from build123d import *

# Parameters (mm, degrees)
BOSS_EXTRUDE1_DEPTH = 10
SKETCH3_R           = 2
BOSS_EXTRUDE2_DEPTH = 10
BOSS_EXTRUDE3_DEPTH = 20
SKETCH6_R           = 2
CUT_EXTRUDE2_DEPTH  = 20
SKETCH4_W           = 40
SKETCH4_H           = 10
CUT_EXTRUDE1_DEPTH  = 31.090136351
FILLET1_R           = 2


with BuildPart() as part:
    # Sketch1 → Boss-Extrude1 (new, symmetric)
    with BuildSketch(Plane(origin=(0, 0, 0), x_dir=(1, 0, 0), z_dir=(0, 1, 0))):
        Polygon((0, -4), (0, 18), (-17.5, 18), (-17.5, 22), (6, 22), (6, -4), align=None)
    extrude(amount=BOSS_EXTRUDE1_DEPTH, both=True)

    # Sketch3 → Boss-Extrude2 (add, symmetric)
    with BuildSketch(Plane(origin=(0, 0, 0), x_dir=(1, 0, 0), z_dir=(0, 1, 0))):
        with BuildLine():
            Line((-3, 4), (0, 4))
            Line((0, 4), (0, -4))
            Line((0, -4), (-3, -4))
            ThreePointArc((-3, -4), (-7, 0), (-3, 4))
        make_face()
        with Locations(Location((-3, 0, 0), (0, 0, 270))):
            Circle(SKETCH3_R, mode=Mode.SUBTRACT)
    extrude(amount=BOSS_EXTRUDE2_DEPTH, both=True)

    # Sketch5 → Boss-Extrude3 (add)
    with BuildSketch(Plane(origin=(0, 10, 0), x_dir=(1, 0, 0), z_dir=(0, 1, 0))):
        with BuildLine():
            Line((0, -4), (10.949747468, -14.949747468))
            ThreePointArc((10.949747468, -14.949747468), (16.606601718, -14.949747468), (16.606601718, -9.292893219))
            Line((16.606601718, -9.292893219), (6, 1.313708499))
            Line((6, 1.313708499), (0, -4))
        make_face()
    extrude(amount=-BOSS_EXTRUDE3_DEPTH)

    # Sketch6 → Cut-Extrude2 (cut)
    with BuildSketch(Plane(origin=(0, 10, 0), x_dir=(1, 0, 0), z_dir=(0, 1, 0))):
        with Locations(Location((13.778174593, -12.121320344, 0), (0, 0, 270))):
            Circle(SKETCH6_R)
    extrude(amount=-CUT_EXTRUDE2_DEPTH, mode=Mode.SUBTRACT)

    # Sketch4 → Cut-Extrude1 (cut, through all)
    with BuildSketch(Plane.XY.offset(-6)):
        with Locations((2.5, 0)):
            Rectangle(SKETCH4_W, SKETCH4_H)
    extrude(amount=CUT_EXTRUDE1_DEPTH, mode=Mode.SUBTRACT)

    # Fillet1
    fillet1_edges = [part.edges().sort_by_distance(p)[0] for p in [
        (6, 7.5, -1.313708499),
        (6, -7.5, -1.313708499),
        (0, -7.5, 4),
        (0, 7.5, 4),
        (0, 0, -18),
        (0, -7.5, -4),
        (0, 7.5, -4),
    ]]
    fillet(fillet1_edges, radius=FILLET1_R)


solid = part.part
Source: CAD feature listing. Evaluate the final solid. Frame: model axes, mm. A direction names the side the tool comes from. Coordinates: 2 decimals unless noted, no trailing zeros. Order: outer loops, then holes, each group sorted by start corner. A loop starts at its lowest first (then second) coordinate and runs counter-clockwise, first axis right, second up. Notation, with made-up numbers: M 63.5,9 L 87.5,9 A21 ccw 87.5,30 Z; hole C 4.5,3 d8. An arc over 180 degrees is marked long. Write each question's results on one line, items separated by ' | '. Start each with the question number.
Item 1: Cut plane A-A (y = -2.5). Return loops of the section in (x, z).
Item 2: Cut plane B-B (z = 0). Return loops of the section in (x, y), and give its area (3 significant figures).
Item 3: Set-up query: faces 5 (the face through (14.38, -7.46, 14.03)), 6 (the face through (-2, 8, 4)), 7 (the face through (11.666, 7.535, 4.353)), 8 (the face through (5, 5, 5)), 9 (the face through (-0.6, 7.46, -4.57)). Return all of +Z, -Z, +X, -X, +Y, -Y with unobstructed straight access to the full face (end or side cutting, diameter ignored); none if empty.
Item 4: Draft query along Z for faces 1 (the face through (0, 0, -11)), 2 (the face through (14.38, 7.54, 14.03)), 3 (the face through (1, -10, -6)), 4 (the face through (3, 0, -6)). Return one class per face: pulls with the +Z half, pulls with the -Z half, needs draft (parallel to the pull), parting line crosses it, or undercut.
Item 5: Line query: probe 1 along Z at (x, y) = (-3, -8.1); probe 2 along Y at (x, z) = (0, 1); probe 3 along Z at (x, y) = (-4.5, -1.5). Output: solid intervals per line, ascending.
Item 6: First-contact query: pin 1 Ø8 at (x, y) = (-12.5, -3.5) entering from +Z; pin 2 Ø1.8 at (x, y) = (1.5, -2.5) entering from +Z; pin 3 Ø10 at (y, z) = (-2.5, 6.5) entering from +X. Flat tips, straight axial feed; report the tip coordinate or a pass-through.
Item 7: Cut plane D-D (y = -8.25). Return loops of the section in (x, z).
Item 8: Cut plane C-C (x = 5.5). Return loops of the section in (y, z), and give its area (3 significant figures).
Checked values:
1) outline: M -17.5,-22 L 6,-22 L 6,-6 L 0,-6 L 0,-16 A2 cw -2,-18 L -17.5,-18 Z
2) outline: M -7,-10 L -5,-10 L -5,-5 L -7,-5 Z; M -7,5 L -5,5 L -5,10 L -7,10 Z; M -1,-10 L 7.31,-10 L 7.31,-5 L -1,-5 Z; M -1,5 L 7.31,5 L 7.31,10 L -1,10 Z | area: 103 mm2
3) face 5: +Y, -Y | face 6: +Z, -X, +Y, -Y | face 7: -Z, +X, +Y, -Y | face 8: +Z, +X, -X | face 9: -X, +Y, -Y
4) face 1: undercut | face 2: undercut | face 3: needs draft | face 4: pulls with the +Z half
5) probe 1: z = -22 to -18, -4 to -2, 2 to 4 | probe 2: y = -10 to -5, 5 to 10 | probe 3: z = -22 to -18
6) pin 1: stops at z = -18 | pin 2: stops at z = -6 | pin 3: stops at x = 17.56
7) outline: M -17.5,-22 L 6,-22 L 6,-2.14 A2 cw 6.59,-0.73 L 16.61,9.29 A4 ccw 10.95,14.95 L 0.59,4.59 A2 cw -0.83,4 L -3,4 A4 ccw -3,-4 L -2,-4 A2 cw 0,-6 L 0,-16 A2 cw -2,-18 L -17.5,-18 Z; hole C -3,0 d4; hole C 13.78,12.12 d4
8) outline: M -10,-22 L 10,-22 L 10,9.5 L 5,9.5 L 5,-6 L -5,-6 L -5,9.5 L -10,9.5 Z | area: 475 mm2
